Verification items for the finished model (mm, model axes). Face numbers are marked on the shaded views. A direction names the side the tool comes from. Round coordinates to 2 decimals unless told otherwise and drop trailing zeros. Write each loop counter-clockwise with the first axis right and the second up, starting at its lowest first coordinate (ties: lowest second). Pieces come first, ordered by that corner, then holes. Notation, with made-up numbers: (-4, 51) -> (55, 51) arc R27 cw to (55, 75) -> close; hole circle Ø6 at (2.5, 53). An arc over 180 degrees is marked (long way). Use CSV: the item, a comma, the result in double quotes.
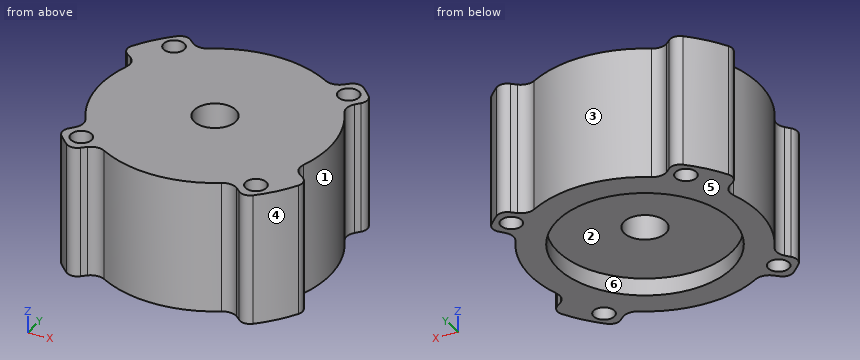
```python
from build123d import *

# Parameters (mm, degrees)
SKETCH1_R               = 3
SKETCH1_R_2             = 1.5
SALIENTE_EXTRUIR1_DEPTH = 19
CROQUIS1_R              = 12.5
CORTAR_EXTRUIR1_DEPTH   = 2.5


with BuildPart() as part:
    # Sketch1 → Saliente-Extruir1 (new body)
    with BuildSketch(Plane.XY):
        with BuildLine():
            ThreePointArc((61.836197312, 3.286280309), (61.020411334, -3.741981398), (63.24135958, -10.459820208))
            ThreePointArc((63.24135958, -10.459820208), (63.516762306, -11.634828053), (63.06603659, -12.754353143))
            ThreePointArc((63.06603659, -12.754353143), (62.779959062, -13.090315668), (62.483190577, -13.416872916))
            ThreePointArc((62.483190577, -13.416872916), (62.077613071, -14.395673215), (62.420017601, -15.398320849))
            ThreePointArc((62.420017601, -15.398320849), (63.193255854, -16.216357175), (64.01129218, -16.989595428))
            ThreePointArc((64.01129218, -16.989595428), (65.013939814, -17.331999958), (65.992740113, -16.926422452))
            ThreePointArc((65.992740113, -16.926422452), (66.319297361, -16.629653967), (66.655259886, -16.343576439))
            ThreePointArc((66.655259886, -16.343576439), (67.774784976, -15.892850723), (68.949792821, -16.168253449))
            ThreePointArc((68.949792821, -16.168253449), (77.335391478, -18.474221551), (85.720990136, -16.168253449))
            ThreePointArc((85.720990136, -16.168253449), (86.89599798, -15.892850723), (88.01552307, -16.343576439))
            ThreePointArc((88.01552307, -16.343576439), (88.351485595, -16.629653967), (88.678042843, -16.926422452))
            ThreePointArc((88.678042843, -16.926422452), (89.656843143, -17.331999958), (90.659490776, -16.989595428))
            ThreePointArc((90.659490776, -16.989595428), (92.842363907, -14.704890816), (94.638151595, -12.104899113))
            ThreePointArc((94.638151595, -12.104899113), (94.770607573, -11.053709999), (94.175376931, -10.17721492))
            ThreePointArc((94.175376931, -10.17721492), (93.818673805, -9.917457245), (93.470537538, -9.646325709))
            ThreePointArc((93.470537538, -9.646325709), (92.802619494, -8.641151304), (92.834585645, -7.434723411))
            ThreePointArc((92.834585645, -7.434723411), (93.650371622, -0.406461703), (91.429423377, 6.311377107))
            ThreePointArc((91.429423377, 6.311377107), (91.154020651, 7.486384951), (91.604746367, 8.605910041))
            ThreePointArc((91.604746367, 8.605910041), (91.890823894, 8.941872566), (92.187592379, 9.268429814))
            ThreePointArc((92.187592379, 9.268429814), (92.593169886, 10.247230114), (92.250765355, 11.249877747))
            ThreePointArc((92.250765355, 11.249877747), (91.477527102, 12.067914073), (90.659490776, 12.841152326))
            ThreePointArc((90.659490776, 12.841152326), (89.656843142, 13.183556857), (88.678042843, 12.77797935))
            ThreePointArc((88.678042843, 12.77797935), (88.351485595, 12.481210865), (88.01552307, 12.195133338))
            ThreePointArc((88.01552307, 12.195133338), (86.89599798, 11.744407622), (85.720990135, 12.019810348))
            ThreePointArc((85.720990135, 12.019810348), (77.335391478, 14.325778449), (68.949792821, 12.019810348))
            ThreePointArc((68.949792821, 12.019810348), (67.774784976, 11.744407622), (66.655259886, 12.195133338))
            ThreePointArc((66.655259886, 12.195133338), (66.319297361, 12.481210865), (65.992740113, 12.77797935))
            ThreePointArc((65.992740113, 12.77797935), (65.013939814, 13.183556857), (64.01129218, 12.841152326))
            ThreePointArc((64.01129218, 12.841152326), (61.828419049, 10.556447714), (60.032631362, 7.956456011))
            ThreePointArc((60.032631362, 7.956456011), (59.900175383, 6.905266897), (60.495406025, 6.028771818))
            ThreePointArc((60.495406025, 6.028771818), (60.852109152, 5.769014143), (61.200245419, 5.497882608))
            ThreePointArc((61.200245419, 5.497882608), (61.868163462, 4.492708203), (61.836197312, 3.286280309))
        make_face()
        with Locations((77.335391478, -2.074221551)):
            Circle(SKETCH1_R, mode=Mode.SUBTRACT)
        with Locations((89.83539148, 10.425778451)):
            Circle(SKETCH1_R_2, mode=Mode.SUBTRACT)
        with Locations((64.835391477, 10.425778451)):
            Circle(SKETCH1_R_2, mode=Mode.SUBTRACT)
        with Locations((89.83539148, -14.574221552)):
            Circle(SKETCH1_R_2, mode=Mode.SUBTRACT)
        with Locations((64.835391477, -14.574221552)):
            Circle(SKETCH1_R_2, mode=Mode.SUBTRACT)
    extrude(amount=SALIENTE_EXTRUIR1_DEPTH)

    # Croquis1 → Cortar-Extruir1 (cut)
    with BuildSketch(Plane(origin=(0, 0, 0), x_dir=(-1, 0, 0), z_dir=(0, 0, -1))):
        with Locations((-77.335391478, -2.074221551)):
            Circle(CROQUIS1_R)
    extrude(amount=-CORTAR_EXTRUIR1_DEPTH, mode=Mode.SUBTRACT)


solid = part.part
```
Q1. Section check B-B (y = -14). Record the cut outline in (x, z).
Filled in:
outline,"(62.14, 0) -> (63.45, 0) -> (63.45, 19) -> (62.14, 19) -> close; (66.22, 0) -> (73.59, 0) -> (73.59, 2.5) -> (81.08, 2.5) -> (81.08, 0) -> (88.45, 0) -> (88.45, 19) -> (66.22, 19) -> close; (91.22, 0) -> (93.39, 0) -> (93.39, 19) -> (91.22, 19) -> close"
Q2. Section check A-A (x = 76.5). Record the cut outline in (y, z), plus the area to 3 significant figures.
Filled in:
outline,"(-18.45, 0) -> (-14.55, 0) -> (-14.55, 2.5) -> (-4.96, 2.5) -> (-4.96, 19) -> (-18.45, 19) -> close; (0.81, 2.5) -> (10.4, 2.5) -> (10.4, 0) -> (14.3, 0) -> (14.3, 19) -> (0.81, 19) -> close"
area,"465 mm²"
Q3. Section check D-D (x = 85). Record the cut outline in (y, z).
Filled in:
outline,"(-16.57, 0) -> (-11.95, 0) -> (-11.95, 2.5) -> (7.8, 2.5) -> (7.8, 0) -> (12.42, 0) -> (12.42, 19) -> (-16.57, 19) -> close"
Q4. Material ranges on L1, parallel to Y at x = 64, z = 17; L2, parallel to X at y = 10, z = 8.75; L3, parallel to Y at x = 90, z = 7.5, recorded low to high.
Filled in:
L1,"-16.98 to -15.82, -13.33 to 9.18, 11.67 to 12.83"
L2,"61.39 to 63.4, 66.27 to 88.4, 91.27 to 92.56"
L3,"-17.3 to -16.07, -13.08 to 8.93, 11.92 to 13.15"
Q5. Mould release check, pull along Y, two halves, no side actions. Record for the marked faces 1, 2, 3 and 4: released by +Y, released by -Y, zero draft, split by the parting line, or undercut.
Filled in:
face 1,"undercut"
face 2,"undercut"
face 3,"released by +Y"
face 4,"released by -Y"
Q6. Access from +Z, -Z, +X, -X, +Y, -Y to the whole of each face (thin tool, end or side, straight path). Record for the marked faces 5 and 6.
Filled in:
face 5,"-Z, +X, -X, +Y, -Y"
face 6,"-Z"
Q7. Section check C-C (y = 5). Record the cut outline in (x, z), plus the area to 3 significant figures.
Filled in:
outline,"(61.64, 0) -> (67.03, 0) -> (67.03, 2.5) -> (87.64, 2.5) -> (87.64, 0) -> (92.13, 0) -> (92.13, 19) -> (61.64, 19) -> close"
area,"528 mm²"
Q8. Go/stop test with flat-tipped pins: P1, Ø1, axis at x = 84.5, y = -2.5, coming from the -Z side; P2, Ø2, axis at y = 7, z = 14, coming from the -X side; P3, Ø3, axis at x = 72.5, z = 3.5, coming from the +Y side; P4, Ø1, axis at y = 3, z = 11, coming from the +X side. Record where each tip stops, or that it passes through.
Filled in:
P1,"z = 2.5"
P2,"x = 59.86"
P3,"y = 13.98"
P4,"x = 93.08"
